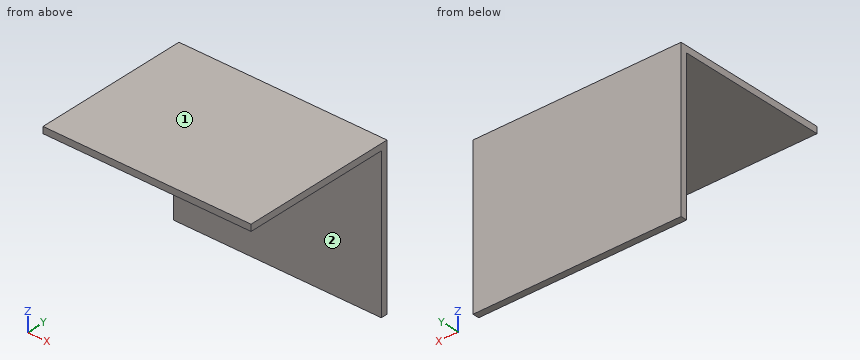
Autodesk Inventor part; units mm, degrees
ref_plane "YZ Plane" through (0, 0, 0) normal (1, 0, 0) x (0, 1, 0)
ref_plane "XZ Plane" through (0, 0, 0) normal (0, 1, 0) x (-1, 0, 0)
ref_plane "XY Plane" through (0, 0, 0) normal (0, 0, 1) x (1, 0, 0)
sketch "Sketch1" plane through (0, 0, 0) normal (1, 0, 0) x (0, 1, 0)
  line L0 (-16.9111, 13.1902) -> (21.1889, 13.1902)
  line L1 (21.1889, 13.1902) -> (21.1889, -24.9098)
  line L2 (21.1889, -24.9098) -> (19.6014, -24.9098)
  line L3 (19.6014, -24.9098) -> (19.6014, 11.6027)
  line L4 (19.6014, 11.6027) -> (-16.9111, 11.6027)
  line L5 (-16.9111, 11.6027) -> (-16.9111, 13.1902)
  point P0 (0, 0)
  dimension "d0" = 38.1
  dimension "d1" = 38.1
  dimension "d2" = 1.5875
  dimension "d3" = 36.5125
  dimension "d4" = 36.5125
extrude "Extrusion1" add sketch "Sketch1" along normal blind 50.8
properties part number "corner piece 2x1.5"
Verification items for the finished model (mm, model axes). Face numbers are marked on the shaded views. A direction names the side the tool comes from. Coordinates: 2 decimals unless noted, no trailing zeros. Loops run counter-clockwise (first coordinate to the right, second up) from the corner with the lowest first, then second, coordinate; pieces in that order, holes last. Notation, with made-up numbers: (-22.75, 59) -> (16.25, 59) arc R17 cw to (16.25, 65) -> close; hole circle Ø11 at (-13.75, -13). An arc over 180 degrees is marked (long way). Answer as a JSON object with one key per item and string values. Group by question number.
Item 1: Depth check by flat-ended pin: pin 1 (18.5 mm diameter, centred on x = 19.5, z = -14.5, fed in from -Y); pin 2 (18.5 mm diameter, centred on x = 29.5, y = 1.5, fed in from -Z). Enter the tip coordinate at first touch or a pass-through.
Item 2: Sectioned sample at B-B on x = 7.5. Record the boundary of the cut face in (y, z).
Item 3: Tool access check on the marked faces 1 and 2. Record the directions out of +Z, -Z, +X, -X, +Y, -Y that give a thin tool (end or side, any length) a straight path to the whole face; none if there is none.
Item 4: Sectioned sample at C-C on y = 8. Record the boundary of the cut face in (x, z), plus the area to 3 significant figures.
Item 5: Scan lines: probe 1 along Z at (x, y) = (30, 7); probe 2 along Y at (x, z) = (3, -8). Record each from-to range of solid material in increasing order.
Item 6: Sectioned sample at A-A on z = 4.5. Record the boundary of the cut face in (x, y).
Evaluation:
{
 "1": {"pin 1": "stops at y = 19.6", "pin 2": "stops at z = 11.6"},
 "2": {"outline": "(-16.91, 11.6) -> (19.6, 11.6) -> (19.6, -24.91) -> (21.19, -24.91) -> (21.19, 13.19) -> (-16.91, 13.19) -> close"},
 "3": {"face 1": "+Z, +X, -X, +Y, -Y", "face 2": "-Z, +X, -X, -Y"},
 "4": {"outline": "(0, 11.6) -> (50.8, 11.6) -> (50.8, 13.19) -> (0, 13.19) -> close", "area": "80.6 mm²"},
 "5": {"probe 1": "z = 11.6 to 13.19", "probe 2": "y = 19.6 to 21.19"},
 "6": {"outline": "(0, 19.6) -> (50.8, 19.6) -> (50.8, 21.19) -> (0, 21.19) -> close"}
}
